Autodesk Fusion 360 part; units mm, degrees
sketch "Sketch1" plane through (0, 0, 0) normal (0, 1, 0) x (1, 0, 0)
  circle A0 centre (26.358, -28.2925) radius 15.5
  line L0 (17.858, -15.331) -> (34.858, -15.331)
  circle A1 centre (26.358, -28.2925) radius 14
  line L1 (17.8035, -17.2101) -> (34.9126, -17.2101)
  line L2 (34.9126, -17.2101) -> (37.1946, -17.2101)
  line L3 (17.8035, -17.2101) -> (15.5215, -17.2101)
  dimension "d1" = 31
  dimension "d2" = 17
  dimension "d3" = 28
extrude "Extrude1" add sketch "Sketch1" along normal blind 15 contours A0 A1 L2 L3 makes body 1
extrude "Extrude2" add sketch "Sketch1" against normal blind 3 contours A0 A1 L2 L3 bodies 1
extrude "Extrude3" add sketch "Sketch1" against normal blind 3 contours A1 L1 bodies 1
sketch "Sketch2" plane through (0, 0, 0) normal (0, 1, 0) x (1, 0, 0)
  circle A0 centre (26.3651, -28.3162) radius 3.5
  dimension "d11" = 7
extrude "Extrude4" add sketch "Sketch2" against normal blind 5 separate body makes body 2
combine "Combine1" operation add target body 2 tool bodies 1
The listing builds one solid part. Answer for the finished solid, in the listing's coordinates (mm). A direction names the side the tool comes from. Coordinates: 2 decimals unless noted, no trailing zeros. Loops run counter-clockwise (first coordinate to the right, second up) from the corner with the lowest first, then second, coordinate; pieces in that order, holes last. Notation, with made-up numbers: (20, 31.5) - (54, 31.5) arc R33 ccw to (54, 59.5) - close; hole circle Ø10 at (-3.75, 36). An arc over 180 degrees is marked (long way). Write item = value, one per line.
1) Section C-C (y = 8.5) is taken. Determine the outline of the cut face in (x, z), plus the area to 3 significant figures.
Responses:
outline = (15.52, 17.21) - (17.8, 17.21) arc R14 cw (long way) to (34.91, 17.21) - (37.19, 17.21) arc R15.5 ccw (long way) to start
area = 107 mm^2
2) Section D-D (z = 25.5) is taken. Determine the outline of the cut face in (x, y).
Responses:
outline = (11.11, -3) - (24.29, -3) - (24.29, -5) - (28.44, -5) - (28.44, -3) - (41.6, -3) - (41.6, 15) - (40.08, 15) - (40.08, 0) - (12.64, 0) - (12.64, 15) - (11.11, 15) - close
3) Section A-A (z = 22.75) is taken. Determine the outline of the cut face in (x, y).
Responses:
outline = (11.88, -3) - (40.83, -3) - (40.83, 15) - (39.21, 15) - (39.21, 0) - (13.5, 0) - (13.5, 15) - (11.88, 15) - close
4) Section B-B (x = 32) is taken. Determine the outline of the cut face in (y, z).
Responses:
outline = (-3, 17.21) - (0, 17.21) - (0, 41.11) - (15, 41.11) - (15, 42.73) - (-3, 42.73) - close
5) Determine the mould class of faces 1 (the face through (26, 0, 30)), 2 (the face through (24, 15, 42.3)), 3 (the face through (26.872, 5.874, 43.784)) for opening direction X: pulls with the +X half, pulls with the -X half, needs draft (parallel to the pull), parting line crosses it, or undercut.
Responses:
face_1 = undercut
face_2 = needs draft
face_3 = parting line crosses it
6) Which of the six approach directions +Z, -Z, +X, -X, +Y, -Y give full straight-line access (tool end or side, diameter ignored) to faces 4 (the face through (25.606, -3.986, 31.733)), 5 (the face through (26.845, 7.395, 42.284)), 6 (the face through (26, -5, 28))?
Responses:
face_4 = -Y
face_5 = +Y
face_6 = +Z, -Z, +X, -X, -Y
7) Each of these flat-tipped pins is pushed along its axis until it touches: P1, Ø2, axis at x = 21.5, y = 7.5, coming from the +Z side; P2, Ø5, axis at y = 12, z = 21, coming from the +X side; P3, Ø8, axis at y = 10, z = 24, coming from the -X side. Where does it stop, or does it pass through?
Responses:
P1 = 43.3
P2 = 41.1
P3 = 10.86
8) Find the intervals of material crossed by line 1 along Y through (x, z) = (39, 20); line 2 along Y through (x, z) = (20, 19.25); line 3 along X through (y, z) = (9.5, 23.25), in increasing order.
Responses:
line_1 = -3 to 15
line_2 = -3 to 0
line_3 = 11.7 to 13.3, 39.42 to 41.01
